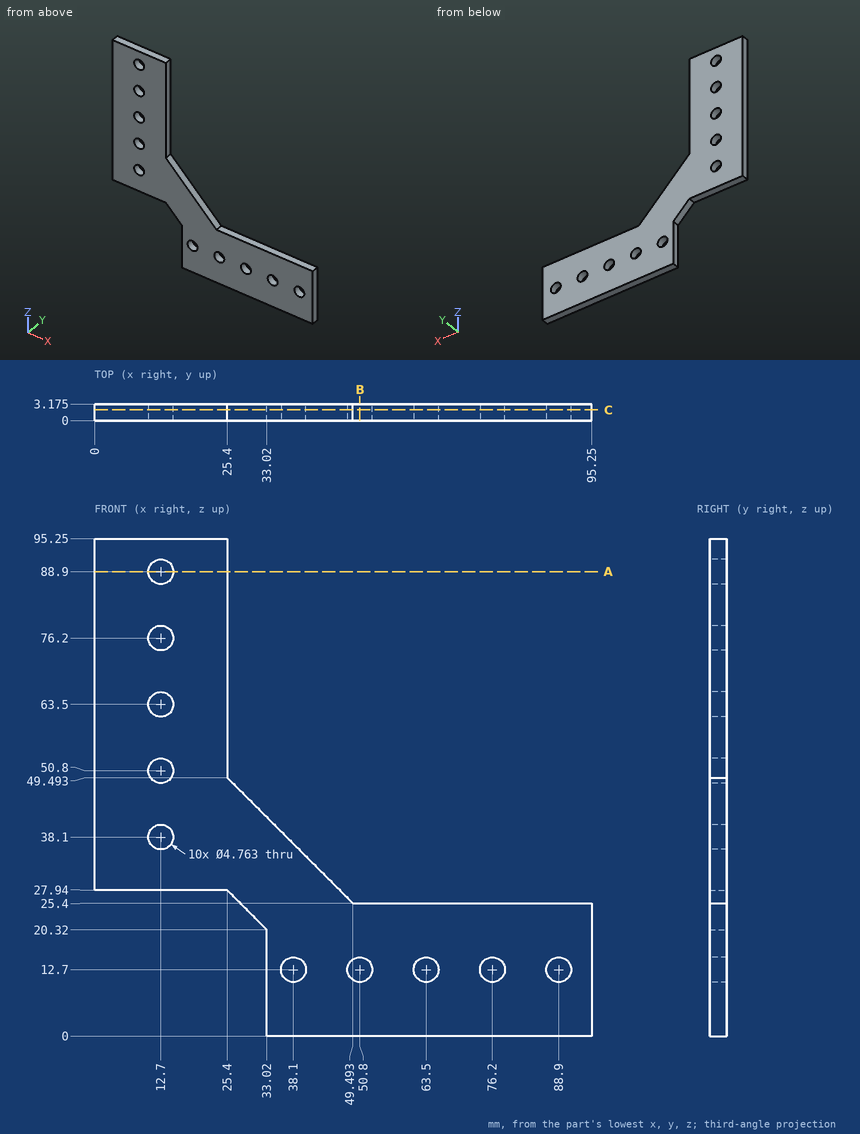
The figure shows three views and two pictorial views of one solid part (mm, origin at its lowest corner). Answer the questions. Give positions to 0.01 mm unless a question says otherwise; leave off trailing zeros. Write each loop counter-clockwise with the first axis right and the second up, starting at its lowest first coordinate (ties: lowest second). Pieces come first, ordered by that corner, then holes. Notation, with made-up numbers: (29.25, 36.5) -> (46.25, 36.5) arc R19 ccw to (46.25, 70.5) -> close; hole circle Ø7 at (48, -20). An arc over 180 degrees is marked (long way). Write each question's results on one line, items separated by ' | '.
1. Find section C-C on y = 2.05. Give the number of separate pieces and of enclosed holes in the cut face, and give its area (3 significant figures).
Data:
separate pieces: 1 | enclosed holes: 10 | area: 3,410 mm^2
2. Straight lines are drawn through the part: L1, parallel to Z at x = 12.7, y = 2.2; L2, parallel to X at y = 2.05, z = 76.2. For each, find the intervals that lie inside material, in ascending order.
Data:
L1: 27.94 to 35.72, 40.48 to 48.42, 53.18 to 61.12, 65.88 to 73.82, 78.58 to 86.52, 91.28 to 95.25 | L2: 0 to 10.32, 15.08 to 25.4
3. Find section A-A on z = 88.9. Determine the outline of the cut face in (x, y) (1 decimal).
Data:
outline: (0, 0) -> (10.3, 0) -> (10.3, 3.2) -> (0, 3.2) -> close; (15.1, 0) -> (25.4, 0) -> (25.4, 3.2) -> (15.1, 3.2) -> close
4. Each of these flat-tipped pins is pushed along its axis until it touches: pin 1 Ø1.5 at (x, y) = (38.5, 2) entering from +Z; pin 2 Ø1 at (x, y) = (10, 2.5) entering from -Z; pin 3 Ø1.6 at (y, z) = (2.5, 68.5) entering from +X; pin 4 Ø4 at (x, z) = (88.9, 12.7) entering from -Y. Where does it stop, or does it pass through?
Data:
pin 1: z = 37.14 | pin 2: z = 27.94 | pin 3: x = 25.4 | pin 4: through
5. Find section B-B on x = 50.8. Determine the outline of the cut face in (y, z) (1 decimal).
Data:
outline: (0, 0) -> (3.2, 0) -> (3.2, 10.3) -> (0, 10.3) -> close; (0, 15.1) -> (3.2, 15.1) -> (3.2, 25.4) -> (0, 25.4) -> close
